Job drawing, mm, ordinate dimensions from the low corner. One solid piece. Round coordinates to 2 decimals unless told otherwise and drop trailing zeros. Loops run counter-clockwise (first coordinate to the right, second up) from the corner with the lowest first, then second, coordinate; pieces in that order, holes last. Notation, with made-up numbers: M 29.5,52.5 L 51.5,52.5 A27 cw 51.5,73.5 Z; hole C -22,59.25 d5. An arc over 180 degrees is marked long. One line per item, written item: value.
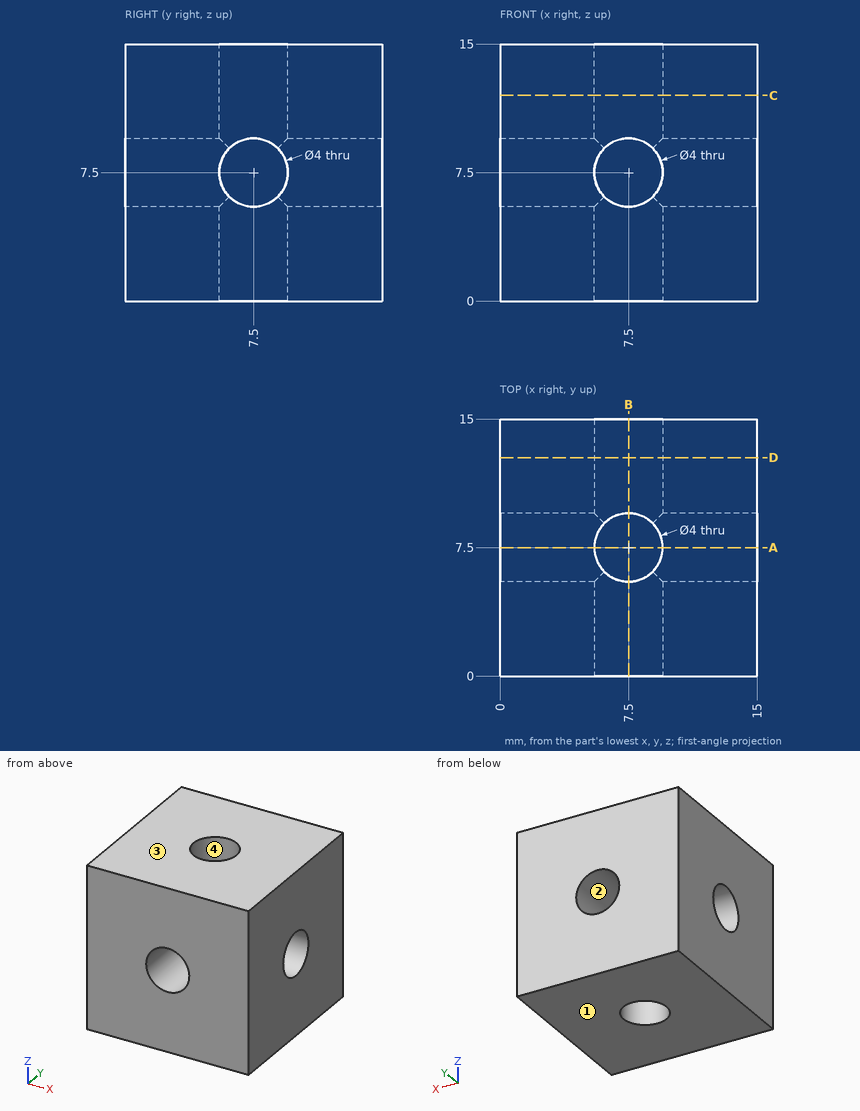
Item 1: Pull direction Z, two halves, no side cores. Call the marked faces 1, 2, 3 and 4: pulls with the +Z half, pulls with the -Z half, needs draft (parallel to the pull), parting line crosses it, or undercut.
Check values:
face 1: pulls with the -Z half
face 2: undercut
face 3: pulls with the +Z half
face 4: needs draft
Item 2: Wall check: line 1 along X through (y, z) = (13.5, 7.5). Give the ranges that are in metal, low to high.
Check values:
line 1: x = 0 to 5.5, 9.5 to 15
Item 3: Slice it at A-A, the plane y = 7.5. Give the cut face in (x, z).
Check values:
outline: M 0,0 L 5.5,0 L 5.5,5.5 L 0,5.5 Z; M 0,9.5 L 5.5,9.5 L 5.5,15 L 0,15 Z; M 9.5,0 L 15,0 L 15,5.5 L 9.5,5.5 Z; M 9.5,9.5 L 15,9.5 L 15,15 L 9.5,15 Z
Item 4: Drop a flat-ended pin along its axis: P1, Ø3.5, axis at x = 7.5, z = 7.5, coming from the -Y side. Give the stop position or say it passes through.
Check values:
P1: passes through
Item 5: Slice it at C-C, the plane z = 12. Give the cut face in (x, y).
Check values:
outline: M 0,0 L 15,0 L 15,15 L 0,15 Z; hole C 7.5,7.5 d4
